Geometry check sheet. Reference: the model listing, model coordinates, mm. A direction names the side the tool comes from. Give positions to 0.01 mm unless a question says otherwise; leave off trailing zeros. Write each loop counter-clockwise with the first axis right and the second up, starting at its lowest first coordinate (ties: lowest second). Pieces come first, ordered by that corner, then holes. Notation, with made-up numbers: (57, 75) -> (94, 75) arc R23 cw to (94, 108) -> close; hole circle Ø2 at (8, -10.5). An arc over 180 degrees is marked (long way). One line per item, written item: value.
from build123d import *

# Parameters (mm, degrees)
BOSS_EXTRUDE1_DEPTH        = 31.75
F_10_CLEARANCE_HOLE1_D     = 5.6134
F_10_CLEARANCE_HOLE1_DEPTH = 25.4
F_10_CLEARANCE_HOLE1_TIP   = 1.686435499
FILLET1_R                  = 1.5875


with BuildPart() as part:
    # Sketch1 → Boss-Extrude1 (new body)
    with BuildSketch(Plane.XY):
        Polygon((0, 0), (0, 19.05), (-3.175, 19.05), (-3.175, 3.175), (-19.05, 3.175), (-19.05, 0), align=None)
    extrude(amount=BOSS_EXTRUDE1_DEPTH)

    # #10 Clearance Hole1
    with Locations(Plane(origin=(0, 3.175, 0), x_dir=(1, 0, 0), z_dir=(0, 1, 0))):
        with Locations((-11.1125, -26.9875), (-11.1125, -4.7625)):
            Hole(F_10_CLEARANCE_HOLE1_D / 2, depth=F_10_CLEARANCE_HOLE1_DEPTH)
            with Locations((0, 0, -(F_10_CLEARANCE_HOLE1_DEPTH + F_10_CLEARANCE_HOLE1_TIP / 2))):  # 118° drill point
                Cone(0, F_10_CLEARANCE_HOLE1_D / 2, F_10_CLEARANCE_HOLE1_TIP, mode=Mode.SUBTRACT)

    # Sketch5 → #10 Clearance Hole2 (revolve, cut)
    with BuildSketch(Plane(origin=(-3.175, 5.6261, 15.875), x_dir=(0, 0, 1), z_dir=(0, 1, 0))):
        Polygon((0, 0), (0, 27.086435499), (2.8067, 25.4), (2.8067, 0), align=None)
    revolve(axis=Axis((-9.525, 5.6261, 15.875), (1, 0, 0)), mode=Mode.SUBTRACT)

    # Fillet1
    fillet1_edges = [part.edges().sort_by_distance(p)[0] for p in [
        (-1.5875, 19.05, 31.75),
        (-19.05, 1.5875, 31.75),
        (-19.05, 1.5875, 0),
        (-1.5875, 19.05, 0),
    ]]
    fillet(fillet1_edges, radius=FILLET1_R)


solid = part.part
1) Sectioned sample at C-C on y = 2. Give the number of separate pieces and of enclosed holes in the cut face, plus the area to 3 significant figures.
Verdict:
separate pieces: 1
enclosed holes: 2
area: 554 mm^2
2) Mould release check, pull along Z, two halves, no side actions. Record for faces 3 (the cylindrical face through (-1.61, 5.5, 13.07)), 4 (the flat face through (-5, 3, 0)), 5 (the cylindrical face through (-18.57, 1.57, 31.3)): released by +Z, released by -Z, zero draft, split by the parting line, or undercut.
Verdict:
face 3: undercut
face 4: released by -Z
face 5: released by +Z
3) Sectioned sample at D-D on x = -15.25. Record the cut outline in (y, z) (3 decimals).
Verdict:
outline: (0, 0) -> (3.175, 0) -> (3.175, 31.75) -> (0, 31.75) -> close
4) Depth check by flat-ended pin: pin 1 Ø1.5 at (y, z) = (10.5, 24) entering from -X (3 decimals); pin 2 Ø3 at (x, z) = (-13, 8.5) entering from +Y (3 decimals). Enter the tip coordinate at first touch or a pass-through.
Verdict:
pin 1: x = -3.175
pin 2: y = 3.175
5) Tool access check on faces 1 (the cylindrical face through (-1.61, 18.57, 31.3)), 2 (the flat face through (-3.175, 11, 16)). Record the directions out of +Z, -Z, +X, -X, +Y, -Y that give a thin tool (end or side, any length) a straight path to the whole face; none if there is none.
Verdict:
face 1: +Z, +X, -X, +Y
face 2: +Z, -Z, -X, +Y
6) Sectioned sample at A-A on z = 16.5. Record the cut outline in (x, y) (3 decimals).
Verdict:
outline: (-19.05, 0) -> (0, 0) -> (0, 2.89) -> (-3.175, 2.89) -> (-3.175, 3.175) -> (-19.05, 3.175) -> close; (-3.175, 8.362) -> (0, 8.362) -> (0, 19.05) -> (-3.175, 19.05) -> close
7) Scan lines: probe 1 along Y at (x, z) = (-14.5, 9.5) (3 decimals); probe 2 along X at (y, z) = (18.25, 20) (3 decimals); probe 3 along Z at (x, y) = (-8.75, 2). Record each from-to range of solid material in increasing order.
Verdict:
probe 1: 0 to 3.175
probe 2: -3.175 to 0
probe 3: 0 to 3.25, 6.28 to 25.47, 28.5 to 31.75
